Read the model definition and answer for the solid it produces. Units are mm, in the model's axes. Face numbers are marked on the shaded views. A direction names the side the tool comes from. Coordinates: 2 decimals unless noted, no trailing zeros. Loops run counter-clockwise (first coordinate to the right, second up) from the corner with the lowest first, then second, coordinate; pieces in that order, holes last. Notation, with made-up numbers: M 32.5,-11.5 L 70.5,-11.5 A22 ccw 70.5,20.5 Z; hole C -32,44.25 d7. An arc over 180 degrees is marked long. Use one line per item in the form item = value. Start each with the question number.
1. The part is cut by section C-C (z = 4.25). Give the vertices of the cut face in (x, y).
2. For a pull along X with two mould halves and no side action, classify the marked faces 3, 4 and 5 as released by +X, released by -X, zero draft, split by the parting line, or undercut.
3. The part is cut by section D-D (x = 7). Give the vertices of the cut face in (y, z).
4. The part is cut by section B-B (y = -11.5). Give the vertices of the cut face in (x, z), plus the area to 3 significant figures.
5. The part is cut by section A-A (z = 10). Give the number of separate pieces and of enclosed holes in the cut face, plus the area to 3 significant figures.
6. A tool of negligible diameter and unlimited length cuts with its end or side. For the marked faces 1 and 2, from which of +Z, -Z, +X, -X, +Y, -Y can it reach the whole face along a straight path? Write none if from no direction.
7. Flat-ended cylindrical pins translate along their axes: pin 1 (12 mm diameter, centred on y = -18, z = 3, fed in from +X); pin 2 (4 mm diameter, centred on x = 9, z = 8, fed in from +Y); pin 3 (4 mm diameter, centred on x = 9, z = 10, fed in from -Y); pin 4 (4 mm diameter, centred on x = 11.5, z = 10, fed in from -Y). Find the tip coordinate at first contact, or state that the pin passes through.
8. Find the intervals of material crossed by probe 1 along X at (y, z) = (1, 3); probe 2 along Z at (x, y) = (10.5, -6.75); probe 3 along Y at (x, z) = (10, 4.75), in increasing order. Write a range as [from, to].
from build123d import *

# Parameters (mm, degrees)
SKETCH1_W           = 20
SKETCH1_H           = 20
BOSS_EXTRUDE1_DEPTH = 4
SKETCH2_R           = 3.7
CUT_EXTRUDE1_DEPTH  = 2.6
SKETCH3_R           = 2.1
CUT_EXTRUDE2_DEPTH  = 29.403520909
SKETCH4_W           = 12
SKETCH4_H           = 4
BOSS_EXTRUDE2_DEPTH = 12
SKETCH7_W           = 20
SKETCH7_H           = 4
BOSS_EXTRUDE3_DEPTH = 5
SKETCH8_W           = 8
SKETCH8_H           = 20
BOSS_EXTRUDE4_DEPTH = 5
SKETCH9_W           = 8
SKETCH9_H           = 20
BOSS_EXTRUDE5_DEPTH = 5
SKETCH10_R          = 1.6
CUT_EXTRUDE5_DEPTH  = 39.288379438
SKETCH11_W          = 30
SKETCH11_H          = 30
CUT_EXTRUDE6_DEPTH  = 6
SKETCH12_R          = 1.45
CUT_EXTRUDE7_DEPTH  = 39.288379438
SKETCH13_W          = 8
SKETCH13_H          = 20
BOSS_EXTRUDE6_DEPTH = 2
SKETCH14_W          = 8
SKETCH14_H          = 20
BOSS_EXTRUDE7_DEPTH = 2
SKETCH15_W          = 16
SKETCH15_H          = 12
CUT_EXTRUDE8_DEPTH  = 37.523964735
FILLET2_R           = 3
FILLET4_R           = 2
FILLET5_START       = -21
FILLET5_DEPTH       = 22
FILLET6_R           = 3
FILLET7_R           = 1
FILLET8_R           = 1


with BuildPart() as part:
    # Sketch1 → Boss-Extrude1 (new body)
    with BuildSketch(Plane(origin=(0, 0, 0), x_dir=(0, 0, -1), z_dir=(1, 0, 0))):
        with Locations((-10, -10)):
            Rectangle(SKETCH1_W, SKETCH1_H)
    extrude(amount=BOSS_EXTRUDE1_DEPTH)

    # Sketch2 → Cut-Extrude1 (cut)
    with BuildSketch(Plane(origin=(4, 0, 0), x_dir=(0, 0, -1), z_dir=(1, 0, 0))):
        with Locations((-10, -10)):
            Circle(SKETCH2_R)
    extrude(amount=-CUT_EXTRUDE1_DEPTH, mode=Mode.SUBTRACT)

    # Sketch3 → Cut-Extrude2 (cut, through all)
    with BuildSketch(Plane(origin=(1.4, 0, 0), x_dir=(0, 0, -1), z_dir=(1, 0, 0))):
        with Locations((-10, -10)):
            Circle(SKETCH3_R)
    extrude(amount=-CUT_EXTRUDE2_DEPTH, mode=Mode.SUBTRACT)

    # Sketch4 → Boss-Extrude2 (add)
    with BuildSketch(Plane(origin=(4, 0, 0), x_dir=(0, 0, -1), z_dir=(1, 0, 0))):
        Polygon((-20, 0), (-20, -20), (-16, -20), (-16, -16), (-16, -4), (-16, 0), align=None)
        with Locations((-10, -18)):
            Rectangle(SKETCH4_W, SKETCH4_H)
        Polygon((-4, -16), (-4, -20), (0, -20), (0, -4), (-4, -4), align=None)
        Polygon((0, 0), (-16, 0), (-16, -4), (-4, -4), (0, -4), align=None)
    extrude(amount=BOSS_EXTRUDE2_DEPTH)

    # Sketch7 → Boss-Extrude3 (add)
    with BuildSketch(Plane(origin=(16, 0, 0), x_dir=(0, 0, -1), z_dir=(1, 0, 0))):
        with Locations((-10, -18)):
            Rectangle(SKETCH7_W, SKETCH7_H)
        with Locations((-10, -2)):
            Rectangle(SKETCH7_W, SKETCH7_H)
    extrude(amount=BOSS_EXTRUDE3_DEPTH)

    # Sketch8 → Boss-Extrude4 (add)
    with BuildSketch(Plane(origin=(0, -20, 0), x_dir=(-1, 0, 0), z_dir=(0, -1, 0))):
        with Locations((-17, -10)):
            Rectangle(SKETCH8_W, SKETCH8_H)
    extrude(amount=BOSS_EXTRUDE4_DEPTH)

    # Sketch9 → Boss-Extrude5 (add)
    with BuildSketch(Plane(origin=(0, 0, 0), x_dir=(1, 0, 0), z_dir=(0, 1, 0))):
        with Locations((17, -10)):
            Rectangle(SKETCH9_W, SKETCH9_H)
    extrude(amount=BOSS_EXTRUDE5_DEPTH)

    # Sketch10 → Cut-Extrude5 (cut, through all)
    with BuildSketch(Plane(origin=(0, 0, 0), x_dir=(-1, 0, 0), z_dir=(0, 0, -1))):
        with Locations(Location((-17, 1, 0), (0, 0, 90))):
            Circle(SKETCH10_R)
        with Locations(Location((-17, -21, 0), (0, 0, 90))):
            Circle(SKETCH10_R)
    extrude(amount=-CUT_EXTRUDE5_DEPTH, mode=Mode.SUBTRACT)

    # Sketch11 → Cut-Extrude6 (cut)
    with BuildSketch(Plane.ZY):
        with Locations((15, -5)):
            Rectangle(SKETCH11_W, SKETCH11_H)
    extrude(amount=-CUT_EXTRUDE6_DEPTH, mode=Mode.SUBTRACT)

    # Sketch12 → Cut-Extrude7 (cut, through all)
    with BuildSketch(Plane(origin=(0, 0, 0), x_dir=(1, 0, 0), z_dir=(0, 1, 0))):
        with Locations(Location((9, -10, 0), (0, 0, 270))):
            Circle(SKETCH12_R)
    extrude(amount=-CUT_EXTRUDE7_DEPTH, mode=Mode.SUBTRACT)

    # Sketch13 → Boss-Extrude6 (add)
    with BuildSketch(Plane.XY.offset(20)):
        with Locations((10, -10)):
            Rectangle(SKETCH13_W, SKETCH13_H)
    extrude(amount=BOSS_EXTRUDE6_DEPTH)

    # Sketch14 → Boss-Extrude7 (add)
    with BuildSketch(Plane(origin=(0, 0, 0), x_dir=(-1, 0, 0), z_dir=(0, 0, -1))):
        with Locations((-10, -10)):
            Rectangle(SKETCH14_W, SKETCH14_H)
    extrude(amount=BOSS_EXTRUDE7_DEPTH)

    # Sketch15 → Cut-Extrude8 (cut, through all)
    with BuildSketch(Plane.ZY.offset(-6)):
        with Locations((10, -10)):
            Rectangle(SKETCH15_W, SKETCH15_H)
    extrude(amount=-CUT_EXTRUDE8_DEPTH, mode=Mode.SUBTRACT)

    # Fillet2
    fillet2_edges = [part.edges().sort_by_distance(p)[0] for p in [
        (21, -16, 10),
        (21, -4, 10),
    ]]
    fillet(fillet2_edges, radius=FILLET2_R)

    # Fillet4
    fillet4_edges = [part.edges().sort_by_distance(p)[0] for p in [
        (21, -25, 10),
        (13, -25, 10),
        (21, 5, 10),
        (13, 5, 10),
    ]]
    fillet(fillet4_edges, radius=FILLET4_R)

    # Fillet5: read off the stored shape, not the designer's step
    # Fillet5 outline → Fillet5 (cut)
    with BuildSketch(Plane(origin=(0, 0, 0), x_dir=(1, 0, 0), z_dir=(0, 1, 0)).offset(FILLET5_START)):
        with BuildLine():
            Line((6, 2), (6, -2))
            ThreePointArc((6, -2), (7.171572875, 0.828427125), (10, 2))
            Line((10, 2), (6, 2))
        make_face()
        with BuildLine():
            ThreePointArc((10, -22), (7.171572875, -20.828427125), (6, -18))
            Line((6, -18), (6, -22))
            Line((6, -22), (10, -22))
        make_face()
    extrude(amount=FILLET5_DEPTH, mode=Mode.SUBTRACT)

    # Fillet6
    # the kernel refuses this fillet: 3 mm, written as the material it takes off along each edge
    with BuildSketch(Plane(origin=(14, -27.071067812, -2), x_dir=(-1, 0, 0), z_dir=(0, 1, 0))) as fillet6_piece_1:
        with BuildLine():
            CenterArc((2.828427125, 3), FILLET6_R, 199.471220634, 70.528779366)
            Line((0, 2), (-0.056568542, 1.98))
            ThreePointArc((-0.056568542, 1.98), (-0.06, 1), (-0.06, 0))
            Line((-0.06, 0), (0, -0.06))
            Line((0, -0.06), (2.828427125, -0.06))
            Line((2.828427125, -0.06), (2.828427125, 0))
        make_face()
    extrude(amount=34.142135624, mode=Mode.SUBTRACT)
    with BuildSketch(Plane(origin=(14, -27.071067812, 22), x_dir=(0, 0, -1), z_dir=(0, 1, 0))) as fillet6_piece_2:
        with BuildLine():
            CenterArc((3, 2.828427125), FILLET6_R, 180, 70.528779366)
            Line((0, 2.828427125), (-0.06, 2.828427125))
            Line((-0.06, 2.828427125), (-0.06, 0))
            Line((-0.06, 0), (0, -0.06))
            ThreePointArc((0, -0.06), (1, -0.06), (1.98, -0.056568542))
            Line((1.98, -0.056568542), (2, 0))
        make_face()
    extrude(amount=34.142135624, mode=Mode.SUBTRACT)

    # Fillet7
    fillet7_edges = [part.edges().sort_by_distance(p)[0] for p in [
        (13, -20, 10),
    ]]
    fillet(fillet7_edges, radius=FILLET7_R)

    # Fillet8
    fillet8_edges = [part.edges().sort_by_distance(p)[0] for p in [
        (13, 0, 10),
    ]]
    fillet(fillet8_edges, radius=FILLET8_R)


solid = part.part
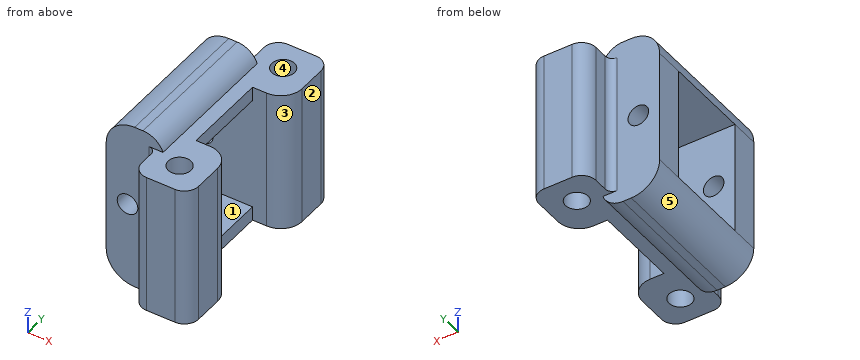
Computed values:
q1.outline = M 6,-20 L 12,-20 A1 cw 13,-21 L 13,-23 A2 ccw 15,-25 L 19,-25 A2 ccw 21,-23 L 21,-19 A3 ccw 18,-16 L 6,-16 Z; M 6,-4 L 18,-4 A3 ccw 21,-1 L 21,3 A2 ccw 19,5 L 15,5 A2 ccw 13,3 L 13,1 A1 cw 12,0 L 6,0 Z; hole C 17,-21 d3.2; hole C 17,1 d3.2
q2.face_3 = released by +X
q2.face_4 = undercut
q2.face_5 = released by -X
q3.outline = M -20,-0.65 L 0,-0.65 L 0,20.65 L -20,20.65 Z; hole M -16,2 L -4,2 L -4,18 L -16,18 Z
q4.outline = M 6,2 A4 ccw 10,-2 L 11.17,-2 A3 ccw 14,0 L 16,0 L 16,2 Z; M 6,18 L 16,18 L 16,20 L 14,20 A3 ccw 11.17,22 L 10,22 A4 ccw Z
q4.area = 62.1 mm²
q5.separate_pieces = 4
q5.enclosed_holes = 2
q5.area = 154 mm²
q6.face_1 = +X, -X
q6.face_2 = +Z, -Z, +X, +Y, -Y
q7.pin_1 = 21
q7.pin_2 = 0
q7.pin_3 = -20
q7.pin_4 = -24.32
q8.probe_1 = [13, 15.4], [18.6, 21]
q8.probe_2 = [-2, 2], [18, 22]
q8.probe_3 = [-20, -16], [-4, 0]
